from build123d import *

# Parameters (mm, degrees)
SALIENTE_EXTRUIR1_DEPTH = 3


with BuildPart() as part:
    # Croquis1 → Saliente-Extruir1 (new body)
    with BuildSketch(Plane(origin=(0, 0, 0), x_dir=(1, 0, 0), z_dir=(0, 1, 0))):
        with BuildLine():
            Line((-59, 0), (-17, 0))
            Line((-17, 0), (-17, 9))
            Line((-17, 9), (-14, 9))
            Line((-14, 9), (-14, 0))
            Line((-14, 0), (-5.5, 0))
            ThreePointArc((-5.5, 0), (0, 5.5), (5.5, 0))
            Line((5.5, 0), (14, 0))
            Line((14, 0), (14, 9))
            Line((14, 9), (17, 9))
            Line((17, 9), (17, 0))
            Line((17, 0), (59, 0))
            Line((59, 0), (59, 20))
            Line((59, 20), (62, 20))
            Line((62, 20), (62, 0))
            Line((62, 0), (70, 0))
            ThreePointArc((70, 0), (0, 70), (-70, 0))
            Line((-70, 0), (-62, 0))
            Line((-62, 0), (-62, 20))
            Line((-62, 20), (-59, 20))
            Line((-59, 20), (-59, 0))
        make_face()
        Polygon((24.748737342, 24.748737342), (29.69848481, 19.798989873), (31.819805153, 21.920310217), (21.920310217, 31.819805153), (19.798989873, 29.69848481), align=None, mode=Mode.SUBTRACT)
        Polygon((-24.748737342, 24.748737342), (-19.798989873, 29.69848481), (-21.920310217, 31.819805153), (-31.819805153, 21.920310217), (-29.69848481, 19.798989873), align=None, mode=Mode.SUBTRACT)
        Polygon((55.861435714, 27.577164466), (27.577164466, 55.861435714), (29.69848481, 57.982756057), (43.840620434, 43.840620434), (57.982756057, 29.69848481), align=None, mode=Mode.SUBTRACT)
        Polygon((-27.577164466, 55.861435714), (-55.861435714, 27.577164466), (-57.982756057, 29.69848481), (-43.840620434, 43.840620434), (-29.69848481, 57.982756057), align=None, mode=Mode.SUBTRACT)
    extrude(amount=SALIENTE_EXTRUIR1_DEPTH)


solid = part.part
The listing builds one solid part. Answer for the finished solid, in the listing's coordinates (mm). A direction names the side the tool comes from. Round coordinates to 2 decimals unless told otherwise and drop trailing zeros. Order: outer loops, then holes, each group sorted by start corner. A loop starts at its lowest first (then second) coordinate and runs counter-clockwise, first axis right, second up. Notation, with made-up numbers: M 31.5,69.5 L 77.5,69.5 A9 ccw 77.5,79.5 Z; hole C 42,58.5 d6. An arc over 180 degrees is marked long. Answer in a Markdown table with one row per item. Add a question column.
1) The part is cut by section D-D on y = 2.1. Count the separate pieces of the cut face and the enclosed holes in it, plus the area to 3 significant figures.
2) Determine the mould class of faces 4 (the face through (-62, 1, -10)), 5 (the face through (41.92, 1.48, -41.52)), 6 (the face through (-38, 1, 0)) for opening direction Z: pulls with the +Z half, pulls with the -Z half, needs draft (parallel to the pull), parting line crosses it, or undercut.
3) Flat-ended cylindrical pins translate along their axes: pin 1 Ø0.9 at (x, y) = (15.5, 2) entering from +Z; pin 2 Ø1.5 at (y, z) = (1, -10) entering from -X; pin 3 Ø0.9 at (x, y) = (-61, 1.5) entering from +Z. Find the tip coordinate at first contact, or state that the pin passes through.
4) The part is cut by section C-C on z = -7. Determine the outline of the cut face in (x, y).
5) The part is cut by section A-A on x = -41.5. Determine the outline of the cut face in (y, z).
6) The part is cut by section B-B on z = -38. Determine the outline of the cut face in (x, y), plus the area to 3 significant figures.
7) Which of the six approach directions +Z, -Z, +X, -X, +Y, -Y give full straight-line access (tool end or side, diameter ignored) to faces 1 (the face through (-41.52, 1.48, -41.92)), 2 (the face through (14, 1, -4)), 3 (the face through (-1, 3, -35))?
8) Consider line 1 along X through (y, z) = (1, -18); line 2 along X through (y, z) = (1.45, -55.5); line 3 along X through (y, z) = (1.05, -8.5). Determine where each line is inside the solid, lowest interval first. Write a range as from..to.
Findings below:
| question | item | result |
|---|---|---|
| 1 | separate pieces | 1 |
| 1 | enclosed holes | 4 |
| 1 | area | 7,150 mm² |
| 2 | face 4 | needs draft |
| 2 | face 5 | undercut |
| 2 | face 6 | pulls with the +Z half |
| 3 | pin 1 | stops at z = -9 |
| 3 | pin 2 | stops at x = -69.39 |
| 3 | pin 3 | stops at z = -20 |
| 4 | outline | M -69.65,0 L -62,0 L -62,3 L -69.65,3 Z; M -59,0 L -17,0 L -17,3 L -59,3 Z; M -14,0 L 14,0 L 14,3 L -14,3 Z; M 17,0 L 59,0 L 59,3 L 17,3 Z; M 62,0 L 69.65,0 L 69.65,3 L 62,3 Z |
| 5 | outline | M 0,-56.37 L 3,-56.37 L 3,-46.18 L 0,-46.18 Z; M 0,-41.94 L 3,-41.94 L 3,0 L 0,0 Z |
| 6 | outline | M -58.79,0 L -49.68,0 L -49.68,3 L -58.79,3 Z; M -45.44,0 L 45.44,0 L 45.44,3 L -45.44,3 Z; M 49.68,0 L 58.79,0 L 58.79,3 L 49.68,3 Z |
| 6 | area | 327 mm² |
| 7 | face 1 | +Y, -Y |
| 7 | face 2 | +Z, +Y, -Y |
| 7 | face 3 | +Z, -Z, +X, -X, +Y |
| 8 | line 1 | x = -67.65..-62, -59..59, 62..67.65 |
| 8 | line 2 | x = -42.66..-32.18, -27.94..27.94, 32.18..42.66 |
| 8 | line 3 | x = -69.48..-62, -59..-17, -14..14, 17..59, 62..69.48 |
